Geometry: final body of the model. Coordinates: model frame, mm. Face numbers are marked on the shaded views. Give positions to 0.01 mm unless a question says otherwise; leave off trailing zeros. Write each loop counter-clockwise with the first axis right and the second up, starting at its lowest first coordinate (ties: lowest second). Pieces come first, ordered by that corner, then holes. Notation, with made-up numbers: M 59,-31 L 112,-31 A27 cw 112,7 Z; hole C 9.5,-14 d11. An arc over 180 degrees is marked long. Use a Markdown table: item, result. Add a question column.
1) Section A-A on x = 5.5. Return the cut outline in (y, z), then the cut area to 3 significant figures.
2) Section D-D on x = 17.5. Return the cut outline in (y, z).
3) Draft query along Z for the marked faces 1, 2, 3 and 4. Return one class per face: +Z half, -Z half, draft (parallel to the pull), parting line (faces both ways), or undercut.
4) Pin query (flat end, axial travel): pin 1 (5 mm diameter, centred on x = -15, z = -8, fed in from -Y); pin 2 (1.5 mm diameter, centred on y = 1, z = -5, fed in from +X); pin 3 (1.5 mm diameter, centred on x = -11.5, y = 0.5, fed in from -Z). Return the tip coordinate at first contact, or that it passes through.
5) Section C-C on z = -8. Return the cut outline in (x, y).
6) Section B-B on y = 2.55. Return the cut outline in (x, z), then the cut area to 3 significant figures.
7) Line query: line 1 (X direction, y = 1.55, z = 8); line 2 (Z direction, x = -15, y = 2.1); line 3 (X direction, y = 0.2, z = 8.75). Output: solid intervals per line, ascending.
```python
from build123d import *

# Parameters (mm, degrees)
SKETCH1_W                = 40
SKETCH1_H                = 25
BOSS_EXTRUDE1_DEPTH      = 3
F_4_0_4_DIAMETER_HOLE1_D = 4
F_4_0_4_DIAMETER_HOLE2_D = 4
SKETCH10_W               = 29
SKETCH10_H               = 14
CUT_EXTRUDE2_DEPTH       = 3
FILLET2_R                = 5


with BuildPart() as part:
    # Sketch1 → Boss-Extrude1 (new body)
    with BuildSketch(Plane(origin=(0, 0, 0), x_dir=(1, 0, 0), z_dir=(0, 1, 0))):
        Rectangle(SKETCH1_W, SKETCH1_H)
    extrude(amount=BOSS_EXTRUDE1_DEPTH)

    # Ø4.0 (4) Diameter Hole1 (through all)
    with Locations(Plane(origin=(0, 3, 0), x_dir=(1, 0, 0), z_dir=(0, 1, 0))):
        with Locations((-15, 8), (15, -8)):
            Hole(F_4_0_4_DIAMETER_HOLE1_D / 2)

    # Ø4.0 (4) Diameter Hole2 (through all)
    with Locations(Plane(origin=(0, 3, 0), x_dir=(1, 0, 0), z_dir=(0, 1, 0))):
        with Locations((-5.5, -7.5), (5.5, -7.5)):
            Hole(F_4_0_4_DIAMETER_HOLE2_D / 2)

    # Sketch10 → Cut-Extrude2 (cut)
    with BuildSketch(Plane(origin=(0, 3, 0), x_dir=(1, 0, 0), z_dir=(0, 1, 0))):
        with Locations((5.5, 5.5)):
            Rectangle(SKETCH10_W, SKETCH10_H)
    extrude(amount=-CUT_EXTRUDE2_DEPTH, mode=Mode.SUBTRACT)

    # Fillet2
    fillet2_edges = [part.edges().sort_by_distance(p)[0] for p in [
        (-9, 1.5, -12.5),
        (20, 1.5, 1.5),
        (-9, 1.5, 1.5),
        (-20, 1.5, -12.5),
        (20, 1.5, 12.5),
        (-20, 1.5, 12.5),
    ]]
    fillet(fillet2_edges, radius=FILLET2_R)


solid = part.part
```
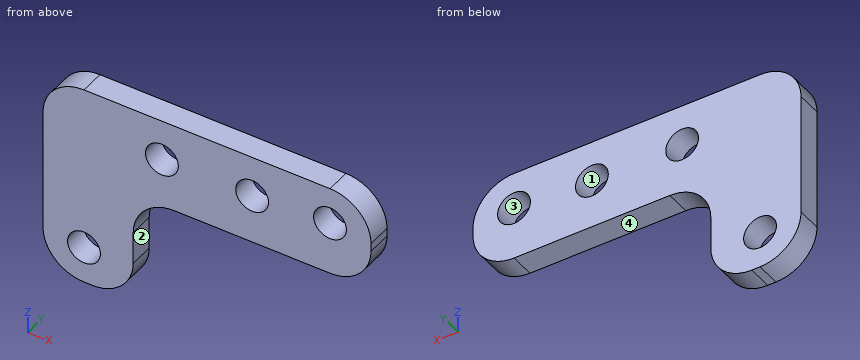
Found:
| question | item | result |
|---|---|---|
| 1 | outline | M 0,1.5 L 3,1.5 L 3,5.5 L 0,5.5 Z; M 0,9.5 L 3,9.5 L 3,12.5 L 0,12.5 Z |
| 1 | area | 21.0 mm² |
| 2 | outline | M 0,2.17 L 3,2.17 L 3,11.83 L 0,11.83 Z |
| 3 | face 1 | undercut |
| 3 | face 2 | draft |
| 3 | face 3 | undercut |
| 3 | face 4 | -Z half |
| 4 | pin 1 | y = 0 |
| 4 | pin 2 | x = -9 |
| 4 | pin 3 | z = -12.18 |
| 5 | outline | M -19.97,0 L -17,0 L -17,3 L -19.97,3 Z; M -13,0 L -9.03,0 L -9.03,3 L -13,3 Z |
| 6 | outline | M -20,-7.5 A5 ccw -15,-12.5 L -14,-12.5 A5 ccw -9,-7.5 L -9,-3.5 A5 cw -4,1.5 L 15,1.5 A5 ccw 20,6.5 L 20,7.5 A5 ccw 15,12.5 L -15,12.5 A5 ccw -20,7.5 Z; hole C -15,-8 d4; hole C -5.5,7.5 d4; hole C 5.5,7.5 d4; hole C 15,8 d4 |
| 6 | area | 522 mm² |
| 7 | line 1 | -19.97 to -7.44, -3.56 to 3.56, 7.44 to 13, 17 to 19.97 |
| 7 | line 2 | -12.5 to -10, -6 to 12.5 |
| 7 | line 3 | -19.84 to -7.06, -3.94 to 3.94, 7.06 to 13.15, 16.85 to 19.84 |
